For this review, take the finished solid that the model builds, in its own axes (mm). Give positions to 0.01 mm unless a question says otherwise; leave off trailing zeros. Order: outer loops, then holes, each group sorted by start corner. A loop starts at its lowest first (then second) coordinate and runs counter-clockwise, first axis right, second up.
from build123d import *

# Parameters (mm, degrees)
ESQUISSE1_R        = 15
ESQUISSE1_R_2      = 6.5
ESQUISSE1_R_3      = 8.5
ESQUISSE1_R_4      = 15.1
ESQUISSE1_R_5      = 7.5
ESQUISSE1_W        = 96
ESQUISSE1_H        = 16
ESQUISSE1_W_2      = 42
ESQUISSE1_H_2      = 12.2
BOSS_EXTRU_1_DEPTH = 10
CONG_1_R           = 10


with BuildPart() as part:
    # Esquisse1 → Boss.-Extru.1 (new body)
    with BuildSketch(Plane.XY):
        Polygon((0, 0), (-1000, 0), (-900, 240), (-810, 240), (-690, 440), (-690, 690), (-610, 690), (-610, 440), (-490, 240), (0, 240), align=None)
        with Locations((-200, 160)):
            Circle(ESQUISSE1_R, mode=Mode.SUBTRACT)
        with Locations((-600, 160)):
            Circle(ESQUISSE1_R, mode=Mode.SUBTRACT)
        with Locations((-393, 170)):
            Circle(ESQUISSE1_R_2, mode=Mode.SUBTRACT)
        with Locations((-393, 42)):
            Circle(ESQUISSE1_R_2, mode=Mode.SUBTRACT)
        with Locations((-673, 89)):
            Circle(ESQUISSE1_R_3, mode=Mode.SUBTRACT)
        with Locations((-500, 180)):
            Circle(ESQUISSE1_R_4, mode=Mode.SUBTRACT)
        with Locations((-650, 650)):
            Circle(ESQUISSE1_R_5, mode=Mode.SUBTRACT)
        with Locations((-650, 610)):
            Circle(ESQUISSE1_R_5, mode=Mode.SUBTRACT)
        with Locations((-650, 570)):
            Circle(ESQUISSE1_R_5, mode=Mode.SUBTRACT)
        with Locations((-650, 530)):
            Circle(ESQUISSE1_R_5, mode=Mode.SUBTRACT)
        with Locations((-650, 490)):
            Circle(ESQUISSE1_R_5, mode=Mode.SUBTRACT)
        with Locations((-650, 450)):
            Circle(ESQUISSE1_R_5, mode=Mode.SUBTRACT)
        with Locations((-57, 133)):
            Rectangle(ESQUISSE1_W, ESQUISSE1_H, mode=Mode.SUBTRACT)
        with Locations((-57, 65)):
            Rectangle(ESQUISSE1_W, ESQUISSE1_H, mode=Mode.SUBTRACT)
        with Locations((-844, 173.9)):
            Rectangle(ESQUISSE1_W_2, ESQUISSE1_H_2, mode=Mode.SUBTRACT)
        with Locations((-679, 173.9)):
            Rectangle(ESQUISSE1_W_2, ESQUISSE1_H_2, mode=Mode.SUBTRACT)
    extrude(amount=BOSS_EXTRU_1_DEPTH)

    # Congé1
    cong_1_edges = [part.edges().sort_by_distance(p)[0] for p in [
        (-900, 240, 5),
        (-810, 240, 5),
        (-690, 440, 5),
        (-690, 690, 5),
        (-610, 690, 5),
        (-610, 440, 5),
        (-490, 240, 5),
        (0, 240, 5),
    ]]
    fillet(cong_1_edges, radius=CONG_1_R)


solid = part.part
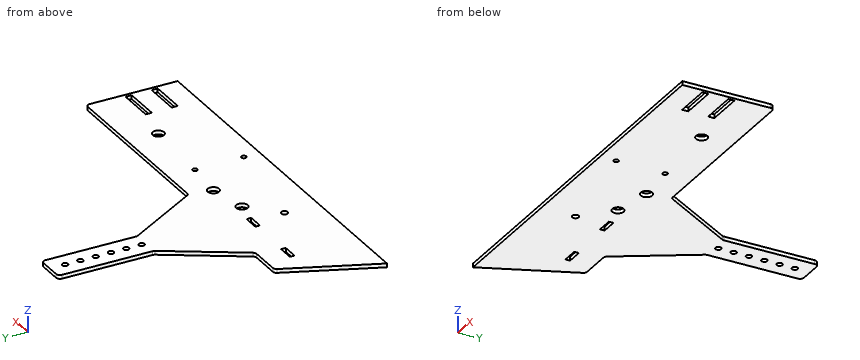
1) To check wall thickness, follow line 1 (Y direction, x = -82, z = 1.5); line 2 (X direction, y = 650, z = 7.25); line 3 (Y direction, x = -125.5, z = 3.5). State the ranges of each line that lie inside material, in increasing order.
Answer sheet:
line 1: y = 0 to 57, 73 to 125, 141 to 240
line 2: x = -690 to -657.5, -642.5 to -610
line 3: y = 0 to 240
2) We need section B-B on z = 4.25. Count the separate pieces of the cut face and the enclosed holes in it, then the cut area to 3 significant figures.
Answer sheet:
separate pieces: 1
enclosed holes: 16
area: 280,000 mm2
3) We need section C-C on x = -756. Give the boundary of the cut face in (y, z).
Answer sheet:
outline: (0, 0) - (330, 0) - (330, 10) - (0, 10) - close
4) We need section A-A on x = -334. Give the boundary of the cut face in (y, z).
Answer sheet:
outline: (0, 0) - (240, 0) - (240, 10) - (0, 10) - close
5) Clearance check with a flat-ended pin moving along its axis: pin 1 (4 mm diameter, centred on y = 572, z = 5.5, fed in from +X). State where the tip first meets the part, or that it passes through.
Answer sheet:
pin 1: stops at x = -610
